from build123d import *

# Parameters (mm, degrees)
ESQUISSE1_W                         = 80
ESQUISSE1_H                         = 53
BOSS_EXTRU_1_DEPTH                  = 19.1
ESQUISSE3_W                         = 77.6
ESQUISSE3_H                         = 50.6
ENL_V_MAT_EXTRU_1_DEPTH             = 16.1
CONG_1_R                            = 4
ESQUISSE9_W                         = 8
ESQUISSE9_H                         = 7
BOSS_EXTRU_2_DEPTH                  = 16.1
ESQUISSE11_R                        = 1.5
ENL_V_MAT_EXTRU_2_DEPTH             = 13.1
ESQUISSE14_W                        = 8
ESQUISSE14_H                        = 7
BOSS_EXTRU_3_DEPTH                  = 16.1
ESQUISSE15_R                        = 1.5
ENL_V_MAT_EXTRU_3_DEPTH             = 13.1
ESQUISSE45_W                        = 8.7
ESQUISSE45_H                        = 12
BOSS_EXTRU_8_DEPTH                  = 0.4
ENL_V_MAT_EXTRU_4_REACH             = 88.412
ESQUISSE18_W                        = 3.5
ESQUISSE18_H                        = 9
ENL_V_MAT_EXTRU_4_DIRECTION_2_DEPTH = 87.412151923
CONG_2_R                            = 0.5
ESQUISSE33_W                        = 4
ESQUISSE33_H                        = 4
BOSS_EXTRU_6_DEPTH                  = 3.9
ESQUISSE35_R                        = 0.75
ENL_V_MAT_EXTRU_6_DEPTH             = 2.9
ENL_V_START                         = -1
ENL_V_MAT_EXTRU_7_DEPTH             = 1
CONG_4_R                            = 0.5
ESQUISSE42_W                        = 11.1
ESQUISSE42_H                        = 10
BOSS_EXTRU_9_DEPTH                  = 1.6
ENL_V_MAT_EXTRU_9_REACH             = 88.783
ESQUISSE40_R                        = 3.2
ENL_V_MAT_EXTRU_9_DIRECTION_2_DEPTH = 87.782601943
CONG_5_R                            = 0.2
ENL_V_MAT_EXTRU_10_REACH            = 71.325
ESQUISSE53_W                        = 8.5
ESQUISSE53_H                        = 4


with BuildPart() as part:
    # Esquisse1 → Boss.-Extru.1 (new body)
    with BuildSketch(Plane.XY):
        Rectangle(ESQUISSE1_W, ESQUISSE1_H)
    extrude(amount=BOSS_EXTRU_1_DEPTH)

    # Esquisse3 → Enlèv. mat.-Extru.1 (cut)
    with BuildSketch(Plane.XY.offset(19.1)):
        Rectangle(ESQUISSE3_W, ESQUISSE3_H)
    extrude(amount=-ENL_V_MAT_EXTRU_1_DEPTH, mode=Mode.SUBTRACT)

    # Congé1
    cong_1_edges = [part.edges().sort_by_distance(p)[0] for p in [
        (38.8, 25.3, 11.05),
        (38.8, -25.3, 11.05),
        (-38.8, -25.3, 11.05),
        (-38.8, 25.3, 11.05),
        (40, -26.5, 9.55),
        (-40, -26.5, 9.55),
        (-40, 26.5, 9.55),
        (40, 26.5, 9.55),
    ]]
    fillet(cong_1_edges, radius=CONG_1_R)

    # Esquisse9 → Boss.-Extru.2 (add)
    with BuildSketch(Plane.XY.offset(3)):
        with Locations((-6.8, -21.8)):
            Rectangle(ESQUISSE9_W, ESQUISSE9_H)
    boss_extru_2 = extrude(amount=BOSS_EXTRU_2_DEPTH)

    # Esquisse11 → Enlèv. mat.-Extru.2 (cut)
    with BuildSketch(Plane.XY.offset(19.1)):
        with Locations((-6.8, -21.8)):
            Circle(ESQUISSE11_R)
    enl_v_mat_extru_2 = extrude(amount=-ENL_V_MAT_EXTRU_2_DEPTH, mode=Mode.SUBTRACT)

    # Symétrie2: Boss.-Extru.2, Enlèv. mat.-Extru.2 across plane
    add(boss_extru_2.mirror(Plane.ZX))
    add(enl_v_mat_extru_2.mirror(Plane.ZX), mode=Mode.SUBTRACT)

    # Esquisse14 → Boss.-Extru.3 (add)
    with BuildSketch(Plane.XY.offset(3)):
        with Locations((30.8, -21.8)):
            Rectangle(ESQUISSE14_W, ESQUISSE14_H)
    boss_extru_3 = extrude(amount=BOSS_EXTRU_3_DEPTH)

    # Esquisse15 → Enlèv. mat.-Extru.3 (cut)
    with BuildSketch(Plane.XY.offset(19.1)):
        with Locations((30.8, -21.8)):
            Circle(ESQUISSE15_R)
    enl_v_mat_extru_3 = extrude(amount=-ENL_V_MAT_EXTRU_3_DEPTH, mode=Mode.SUBTRACT)

    # Symétrie3: Boss.-Extru.3, Enlèv. mat.-Extru.3 across plane
    add(boss_extru_3.mirror(Plane.ZX))
    add(enl_v_mat_extru_3.mirror(Plane.ZX), mode=Mode.SUBTRACT)

    # Esquisse45 → Boss.-Extru.8 (add)
    with BuildSketch(Plane(origin=(40, 0, 0), x_dir=(0, 0, -1), z_dir=(1, 0, 0))):
        with Locations((-14.75, 0)):
            Rectangle(ESQUISSE45_W, ESQUISSE45_H)
    extrude(amount=BOSS_EXTRU_8_DEPTH)

    # Esquisse18 → Enlèv. mat.-Extru.4 (cut, up to next)
    with BuildSketch(Plane(origin=(40, 0, 0), x_dir=(0, 0, -1), z_dir=(1, 0, 0)), mode=Mode.PRIVATE) as enl_v_mat_extru_4_sk1:
        with Locations((-14.75, 0)):
            Rectangle(ESQUISSE18_W, ESQUISSE18_H)
    enl_v_mat_extru_4_tool1 = extrude(enl_v_mat_extru_4_sk1.sketch, amount=-ENL_V_MAT_EXTRU_4_REACH, mode=Mode.PRIVATE) & part.part
    add(enl_v_mat_extru_4_tool1.solids().sort_by_distance((40, 0, 14.75))[0], mode=Mode.SUBTRACT)

    # Esquisse18 → Enlèv. mat.-Extru.4 direction 2 (cut)
    with BuildSketch(Plane(origin=(40, 0, 0), x_dir=(0, 0, -1), z_dir=(1, 0, 0))):
        with Locations((-14.75, 0)):
            Rectangle(ESQUISSE18_W, ESQUISSE18_H)
    extrude(amount=ENL_V_MAT_EXTRU_4_DIRECTION_2_DEPTH, mode=Mode.SUBTRACT)

    # Congé2
    cong_2_edges = [part.edges().sort_by_distance(p)[0] for p in [
        (39.6, -4.5, 13),
        (39.6, 4.5, 13),
        (39.6, 4.5, 16.5),
        (39.6, -4.5, 16.5),
    ]]
    fillet(cong_2_edges, radius=CONG_2_R)

    # Esquisse33 → Boss.-Extru.6 (add)
    with BuildSketch(Plane.XY.offset(3)):
        with Locations((12, -18.3)):
            Rectangle(ESQUISSE33_W, ESQUISSE33_H)
    boss_extru_6 = extrude(amount=BOSS_EXTRU_6_DEPTH)

    # Esquisse35 → Enlèv. mat.-Extru.6 (cut)
    with BuildSketch(Plane.XY.offset(6.9)):
        with Locations((12, -18.3)):
            Circle(ESQUISSE35_R)
    enl_v_mat_extru_6 = extrude(amount=-ENL_V_MAT_EXTRU_6_DEPTH, mode=Mode.SUBTRACT)

    # Symétrie4: Boss.-Extru.6, Enlèv. mat.-Extru.6 across plane
    add(boss_extru_6.mirror(Plane.ZX))
    add(enl_v_mat_extru_6.mirror(Plane.ZX), mode=Mode.SUBTRACT)

    # Esquisse38 → Enlèv. mat.-Extru.7 (cut)
    with BuildSketch(Plane.XY.offset(3).offset(ENL_V_START)):
        with BuildLine():
            Line((-10.8, -25.3), (-10.8, 25.3))
            Line((-10.8, 25.3), (-34.8, 25.3))
            ThreePointArc((-34.8, 25.3), (-37.628427125, 24.128427125), (-38.8, 21.3))
            Line((-38.8, 21.3), (-38.8, -21.3))
            ThreePointArc((-38.8, -21.3), (-37.628427125, -24.128427125), (-34.8, -25.3))
            Line((-34.8, -25.3), (-10.8, -25.3))
        make_face()
    extrude(amount=ENL_V_MAT_EXTRU_7_DEPTH, mode=Mode.SUBTRACT)

    # Congé4
    cong_4_edges = [part.edges().sort_by_distance(p)[0] for p in [
        (-10.8, 0, 2),
    ]]
    fillet(cong_4_edges, radius=CONG_4_R)

    # Esquisse42 → Boss.-Extru.9 (add)
    with BuildSketch(Plane(origin=(-38.8, 0, 0), x_dir=(0, 0, -1), z_dir=(1, 0, 0))):
        with Locations((-13.55, 0)):
            Rectangle(ESQUISSE42_W, ESQUISSE42_H)
    extrude(amount=-BOSS_EXTRU_9_DEPTH)

    # Esquisse40 → Enlèv. mat.-Extru.9 (cut, up to next)
    with BuildSketch(Plane.ZY.offset(40), mode=Mode.PRIVATE) as enl_v_mat_extru_9_sk1:
        with Locations((13.55, 0)):
            Circle(ESQUISSE40_R)
    enl_v_mat_extru_9_tool1 = extrude(enl_v_mat_extru_9_sk1.sketch, amount=-ENL_V_MAT_EXTRU_9_REACH, mode=Mode.PRIVATE) & part.part
    add(enl_v_mat_extru_9_tool1.solids().sort_by_distance((-40, 0, 13.55))[0], mode=Mode.SUBTRACT)

    # Esquisse40 → Enlèv. mat.-Extru.9 direction 2 (cut)
    with BuildSketch(Plane.ZY.offset(40)):
        with Locations((13.55, 0)):
            Circle(ESQUISSE40_R)
    extrude(amount=ENL_V_MAT_EXTRU_9_DIRECTION_2_DEPTH, mode=Mode.SUBTRACT)

    # Congé5
    cong_5_edges = [part.edges().sort_by_distance(p)[0] for p in [
        (34.8, -21.8, 19.1),
        (34.8, 21.8, 19.1),
    ]]
    fillet(cong_5_edges, radius=CONG_5_R)

    # Esquisse53 → Enlèv. mat.-Extru.10 (cut, up to next)
    with BuildSketch(Plane(origin=(0, -26.5, 0), x_dir=(-1, 0, 0), z_dir=(0, -1, 0)), mode=Mode.PRIVATE) as enl_v_mat_extru_10_sk1:
        with Locations((15.05, -14.6)):
            Rectangle(ESQUISSE53_W, ESQUISSE53_H)
    enl_v_mat_extru_10_tool1 = extrude(enl_v_mat_extru_10_sk1.sketch, amount=-ENL_V_MAT_EXTRU_10_REACH, mode=Mode.PRIVATE) & part.part
    add(enl_v_mat_extru_10_tool1.solids().sort_by_distance((-15.05, -26.5, 14.6))[0], mode=Mode.SUBTRACT)


solid = part.part
Build history of the part. All positions in model axes, mm. A direction names the side the tool comes from. Round coordinates to 2 decimals unless told otherwise and drop trailing zeros. Write each loop counter-clockwise with the first axis right and the second up, starting at its lowest first coordinate (ties: lowest second). Pieces come first, ordered by that corner, then holes. Notation, with made-up numbers: M 86,59.25 L 144,59.25 A22 ccw 144,82.25 Z; hole C 53,-17.5 d11. An arc over 180 degrees is marked long. Answer as a JSON object with one key per item and string values. Group by question number.
(1) Cut at D-D (y = 14). Give the cut face in (x, z), and give its area (3 significant figures).
(2) Flat gauge pins, fed straight in: pin 1 (1.5 mm diameter, centred on y = -1, z = 13.5, fed in from -X); pin 2 (5 mm diameter, centred on y = 8.5, z = 12.5, fed in from -X); pin 3 (1.5 mm diameter, centred on x = -4.5, y = 1, fed in from +Z). Where does each tip first touch, or does it go through?
(3) Cut at A-A (y = 0). Give the cut face in (x, z), and give its area (3 significant figures).
(4) Mould opens along X. For faces 4 (the cylindrical face through (-38.859, 25.297, 9.684)), 5 (the flat face through (-1, 0, 0)), 6 (the flat face through (-2.8, 22, 11)), 7 (the flat face through (12, -20.3, 5)) say: pulls with the +X half, pulls with the -X half, needs draft (parallel to the pull), parting line crosses it, or undercut.
(5) Drill centre lines: L1, parallel to Y at x = -6.8, z = 15.75; L2, parallel to Y at x = 12, z = 5.3; L3, parallel to X at y = 20, z = 18.25. Where is each one in solid material? Low to high.
(6) Cut at B-B (x = -14.5). Give the cut face in (y, z), and give its area (3 significant figures).
(7) Cut at C-C (x = 16). Give the cut face in (y, z).
(8) Which spindle directions (+Z, -Z, +X, -X, +Y, -Y) get a long thin tool onto all of the face, cutting with end or side? Do faces 1 (the flat face through (40, 0, 16.5)), 2 (the cylindrical face through (38.797, -25.359, 9.684)), 3 (the flat face through (12, -16.3, 5)). Say none if no direction does.
Responses:
{
 "1": {"outline": "M -40,0 L 40,0 L 40,19.1 L 38.8,19.1 L 38.8,3 L -10.8,3 L -10.8,2.5 A0.5 cw -11.3,2 L -38.8,2 L -38.8,19.1 L -40,19.1 Z", "area": "251 mm2"},
 "2": {"pin 1": "stops at x = 38.8", "pin 2": "stops at x = -40", "pin 3": "stops at z = 3"},
 "3": {"outline": "M -40.4,8 L -40,8 L -40,0 L 40,0 L 40,10.4 L 40.4,10.4 L 40.4,13 L 38.8,13 L 38.8,3 L -10.8,3 L -10.8,2.5 A0.5 cw -11.3,2 L -38.8,2 L -38.8,10.35 L -40.4,10.35 Z; M -40.4,16.75 L -38.8,16.75 L -38.8,19.1 L -40.4,19.1 Z; M 38.8,16.5 L 40.4,16.5 L 40.4,19.1 L 38.8,19.1 Z", "area": "243 mm2"},
 "4": {"face 4": "pulls with the -X half", "face 5": "needs draft", "face 6": "undercut", "face 7": "undercut"},
 "5": {"L1": "y = -26.5 to -23.3, -20.3 to -18.3, 18.3 to 20.3, 23.3 to 26.5", "L2": "y = -26.5 to -25.3, -20.3 to -19.05, -17.55 to -16.3, 16.3 to 17.55, 19.05 to 20.3, 25.3 to 26.5", "L3": "x = -40 to -38.8, -10.8 to -2.8, 26.8 to 34.8, 38.8 to 40"},
 "6": {"outline": "M -26.5,0 L 26.5,0 L 26.5,19.1 L 25.3,19.1 L 25.3,2 L -25.3,2 L -25.3,12.6 L -26.5,12.6 Z; M -26.5,16.6 L -25.3,16.6 L -25.3,19.1 L -26.5,19.1 Z", "area": "142 mm2"},
 "7": {"outline": "M -26.5,0 L 26.5,0 L 26.5,19.1 L 25.3,19.1 L 25.3,3 L -25.3,3 L -25.3,19.1 L -26.5,19.1 Z"},
 "8": {"face 1": "+X", "face 2": "+Z, -Z, +X, -Y", "face 3": "+Z"}
}
